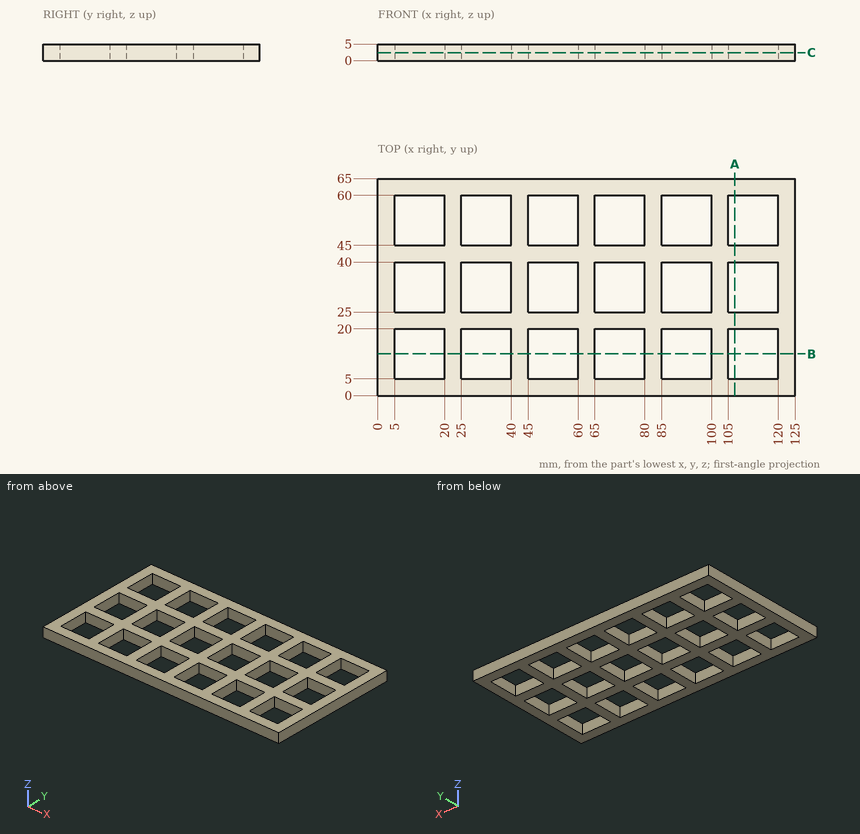
Study the drawing (mm; zero at the part's minimum x, y, z) and answer. Round coordinates to 2 decimals unless told otherwise and drop trailing zeros. Order: outer loops, then holes, each group sorted by start corner. A loop starts at its lowest first (then second) coordinate and runs counter-clockwise, first axis right, second up. Notation, with made-up numbers: (5.25, 87.5) -> (10.25, 87.5) arc R35 cw to (10.25, 125.5) -> close; hole circle Ø9 at (24, 89.5). An arc over 180 degrees is marked (long way). Answer as CSV lines item,"result". Start each with the question number.
(1) Find the intervals of material crossed by probe 1 along Y at (x, z) = (75, 3.55), in increasing order. Write a range as from..to.
(2) Flat-ended cylindrical pins translate along their axes: pin 1 Ø1.5 at (x, z) = (73, 2) entering from -Y; pin 2 Ø10 at (x, y) = (74.5, 13.5) entering from -Z. Find the tip coordinate at first contact, or state that the pin passes through.
(3) The part is cut by section C-C (z = 2.45). Count the separate pieces of the cut face and the enclosed holes in it, then the cut area to 4 significant figures.
(4) The part is cut by section A-A (x = 107). Determine the outline of the cut face in (y, z), then the cut area to 3 significant figures.
(5) The part is cut by section B-B (y = 12.5). Determine the outline of the cut face in (x, z).
Evaluation:
1,probe 1,"0..5, 20..25, 40..45, 60..65"
2,pin 1,"y = 0"
2,pin 2,"through"
3,separate pieces,"1"
3,enclosed holes,"18"
3,area,"4,075 mm²"
4,outline,"(0, 0) -> (5, 0) -> (5, 5) -> (0, 5) -> close; (20, 0) -> (25, 0) -> (25, 5) -> (20, 5) -> close; (40, 0) -> (45, 0) -> (45, 5) -> (40, 5) -> close; (60, 0) -> (65, 0) -> (65, 5) -> (60, 5) -> close"
4,area,"100 mm²"
5,outline,"(0, 0) -> (5, 0) -> (5, 5) -> (0, 5) -> close; (20, 0) -> (25, 0) -> (25, 5) -> (20, 5) -> close; (40, 0) -> (45, 0) -> (45, 5) -> (40, 5) -> close; (60, 0) -> (65, 0) -> (65, 5) -> (60, 5) -> close; (80, 0) -> (85, 0) -> (85, 5) -> (80, 5) -> close; (100, 0) -> (105, 0) -> (105, 5) -> (100, 5) -> close; (120, 0) -> (125, 0) -> (125, 5) -> (120, 5) -> close"
